from build123d import *

# Parameters (mm, degrees)
F1_DEPTH      = 10
F3_W          = 12
F3_H          = 23
F3_R          = 4.05
F4_DEPTH      = 80
F5_W          = 2
F5_H          = 39.0547718853
F6_DEPTH      = 80
F7_W          = 11
F7_H          = 1
F7_W_2        = 13
F7_H_2        = 20
F7_R          = 3
F8_DEPTH      = 25
F10_DEPTH     = 2.5
F11_T1_DEPTH  = 87.5
F11_T3_DEPTH  = 54
F11_T5_DEPTH  = 27.5
F11_T10_DEPTH = 85.7106781187
F11_T16_DEPTH = 85.7106781187


# Not quite as in the source:
# - a fillet or chamfer that OpenCascade refuses, or shapes differently, is made with other operations: its cross-section is extruded or revolved along the edge and cut away or added


with BuildPart() as f1:
    # F0 (on Top) → F1 (new body)
    with BuildSketch(Plane.XY):
        Polygon((6, 22), (0, 22), (-6, 22), (-6, 12), (-90, 12), (-90, 0), (-6, 0), (-6, -80), (6, -80), (6, 0), (90, 0), (90, 12), (6, 12), align=None)
    extrude(amount=F1_DEPTH)

    # F3 (on face) → F4 (join)
    with BuildSketch(Plane.XY.offset(10)):
        with Locations((0, 11.5)):
            Rectangle(F3_W, F3_H)
        with Locations((0, 6)):
            Circle(F3_R, mode=Mode.SUBTRACT)
    extrude(amount=F4_DEPTH)

    # F5 (on face) → F6 (cut, through all)
    with BuildSketch(Plane.XY.offset(10)):
        with Locations((0, 25.7887821645)):
            Rectangle(F5_W, F5_H)
    extrude(amount=F6_DEPTH, mode=Mode.SUBTRACT)

    # F7 (on face) → F8 (cut)
    with BuildSketch(Plane(origin=(-6, 0, 0), x_dir=(0, -1, 0), z_dir=(-1, 0, 0))):
        with Locations((-17.5, 10.5)):
            Rectangle(F7_W, F7_H)
        with Locations((-16.5, 41)):
            Rectangle(F7_W_2, F7_H_2)
        with Locations((-17, 21)):
            Circle(F7_R)
        with Locations((-17, 78)):
            Circle(F7_R)
        with Locations((-17, 63)):
            Circle(F7_R)
    extrude(amount=-F8_DEPTH, mode=Mode.SUBTRACT)

    # F9 (on Right) → F10 (join, symmetric)
    with BuildSketch(Plane.YZ):
        Polygon((0, 10), (0, 60), (-50, 10), align=None)
    extrude(amount=F10_DEPTH, both=True)

    # F11: fillet of radius 3 on 8 edges, made by hand

    # F11_s2 → F11_t1 (cut)
    with BuildSketch(Plane.XY.offset(10)):
        with BuildLine():
            ThreePointArc((-6, 3), (-5.1213203436, 0.8786796564), (-3, 0))
            Line((-3, 0), (-6, 0))
            Line((-6, 0), (-6, 3))
        make_face()
        with BuildLine():
            ThreePointArc((6, 3), (5.1213203436, 0.8786796564), (3, 0))
            Line((3, 0), (6, 0))
            Line((6, 0), (6, 3))
        make_face()
    extrude(amount=F11_T1_DEPTH, mode=Mode.SUBTRACT)

    # F11_s4 → F11_t3 (cut)
    with BuildSketch(Plane.XY.offset(43.5)):
        with BuildLine():
            ThreePointArc((-3, 23), (-5.1213203436, 22.1213203436), (-6, 20))
            Line((-6, 20), (-6, 23))
            Line((-6, 23), (-3, 23))
        make_face()
        with BuildLine():
            ThreePointArc((6, 20), (5.1213203436, 22.1213203436), (3, 23))
            Line((3, 23), (6, 23))
            Line((6, 23), (6, 20))
        make_face()
    extrude(amount=F11_T3_DEPTH, mode=Mode.SUBTRACT)

    # F11_s6 → F11_t5 (cut)
    with BuildSketch(Plane.XY.offset(11)):
        with BuildLine():
            ThreePointArc((6, 20), (5.1213203436, 22.1213203436), (3, 23))
            Line((3, 23), (6, 23))
            Line((6, 23), (6, 20))
        make_face()
        with BuildLine():
            ThreePointArc((-3, 23), (-5.1213203436, 22.1213203436), (-6, 20))
            Line((-6, 20), (-6, 23))
            Line((-6, 23), (-3, 23))
        make_face()
    extrude(amount=F11_T5_DEPTH, mode=Mode.SUBTRACT)


with BuildPart() as f11_tool8:
    # F11_s9 → F11_t10 (new body)
    with BuildSketch(Plane(origin=(0, 35.3033008589, 35.3033008589), x_dir=(1, 0, 0), z_dir=(0, -0.7071067812, -0.7071067812))):
        with BuildLine():
            ThreePointArc((-2.5, 39.4264068712), (-1.6213203436, 41.5477272148), (0.5, 42.4264068712))
            Line((0.5, 42.4264068712), (-2.5, 42.4264068712))
            Line((-2.5, 42.4264068712), (-2.5, 39.4264068712))
        make_face()
    extrude(amount=F11_T10_DEPTH)

    split(bisect_by=Plane.XY.offset(10), keep=Keep.TOP)

    split(bisect_by=Plane.XZ, keep=Keep.TOP)


with BuildPart() as f1_1:
    add(f1.part)

    # F11_t7: cut F11_tool8
    add(f11_tool8.part, mode=Mode.SUBTRACT)


with BuildPart() as f11_tool14:
    # F11_s15 → F11_t16 (new body)
    with BuildSketch(Plane(origin=(0, 35.3033008589, 35.3033008589), x_dir=(1, 0, 0), z_dir=(0, -0.7071067812, -0.7071067812))):
        with BuildLine():
            ThreePointArc((-0.5, 42.4264068712), (1.6213203436, 41.5477272148), (2.5, 39.4264068712))
            Line((2.5, 39.4264068712), (2.5, 42.4264068712))
            Line((2.5, 42.4264068712), (-0.5, 42.4264068712))
        make_face()
    extrude(amount=F11_T16_DEPTH)

    split(bisect_by=Plane.XY.offset(10), keep=Keep.TOP)

    split(bisect_by=Plane.XZ, keep=Keep.TOP)


with BuildPart() as f1_2:
    add(f1_1.part)

    # F11_t13: cut F11_tool14
    add(f11_tool14.part, mode=Mode.SUBTRACT)


solid = f1_2.part
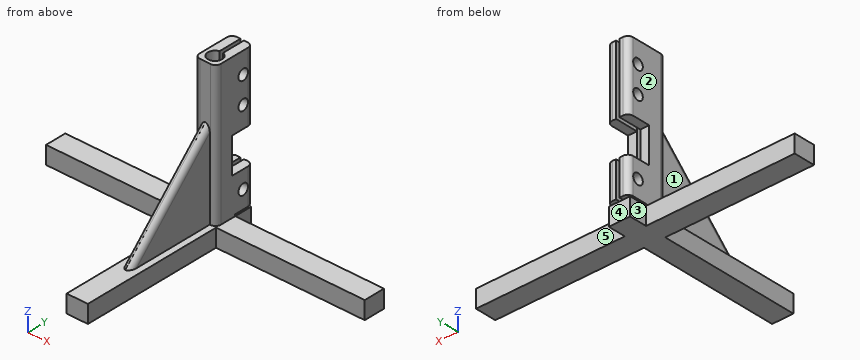
Could you check a few things on this model? Use its own coordinates, in mm. Face numbers are marked on the shaded views. A direction names the side the tool comes from. Coordinates: 2 decimals unless noted, no trailing zeros. Order: outer loops, then holes, each group sorted by start corner. A loop starts at its lowest first (then second) coordinate and runs counter-clockwise, first axis right, second up.
Q1. Please list where these lines run through material, in increasing order: L1, parallel to Z at x = 4.05, y = 17; L2, parallel to Y at x = 2.9, z = 21; L3, parallel to X at y = 16.5, z = 27.
Q2. Will these pins go through, and if not, where does the flat tip stop? pin 1 (2 mm diameter, centred on y = -24.5, z = 35, fed in from -X); pin 2 (9.5 mm diameter, centred on y = 17, z = 21, fed in from +X); pin 3 (5 mm diameter, centred on y = 12.5, z = 49.5, fed in from -X); pin 4 (6.5 mm diameter, centred on y = 19, z = 34.5, fed in from +X).
Q3. Which directions (+Z, -Z, +X, -X, +Y, -Y) give clear straight access to the entire face, cutting with the end or side of a thin tool? Please do the marked faces 1, 2, 3, 4 and 5.
Q4. Suppose I cut it at B-B on z = 70.5. Please give me the cut outline in (x, y), and give its area (3 significant figures).
Q5. Suppose I cut it at C-C on x = -35.5. Please give me the cut outline in (y, z).
Q6. Suppose I cut it at A-A on y = 6. Please give me the cut outline in (x, z).
Q7. Suppose I cut it at D-D on y = -67.5. Please give me the cut outline in (x, z), and give its area (3 significant figures).
Answer:
1. L1: z = 0 to 10, 11 to 18, 24 to 31, 51 to 60, 66 to 75, 81 to 90
1. L2: y = 0 to 3.17, 8.83 to 14, 20 to 23
1. L3: x = -6 to -1, 1 to 6
2. pin 1: stops at x = -2.01
2. pin 2: stops at x = 6
2. pin 3: stops at x = -6
2. pin 4: passes through
3. face 1: +Z, -X, -Y
3. face 2: +Z, -X, +Y, -Y
3. face 3: +Z, -Z, -X, +Y
3. face 4: -Z, +X, -X, +Y
3. face 5: +Z, -Z, +X, +Y
4. outline: (-6, 3) arc R3 ccw to (-3, 0) - (3, 0) arc R3 ccw to (6, 3) - (6, 20) arc R3 ccw to (3, 23) - (1, 23) - (1, 9.92) arc R4.05 cw (long way) to (-1, 9.92) - (-1, 23) - (-3, 23) arc R3 ccw to (-6, 20) - close
4. area: 191 mm2
5. outline: (0, 0) - (12, 0) - (12, 10) - (0, 10) - close
6. outline: (-90, 0) - (90, 0) - (90, 10) - (6, 10) - (6, 90) - (4.05, 90) - (4.05, 10) - (-4.05, 10) - (-4.05, 90) - (-6, 90) - (-6, 10) - (-90, 10) - close
7. outline: (-6, 0) - (6, 0) - (6, 10) - (-6, 10) - close
7. area: 120 mm2
